Check sheet for the drawn part. Datum: minimum x, y, z corner. Units: mm. A direction names the side the tool comes from. Round coordinates to 2 decimals unless told otherwise and drop trailing zeros. Write each loop counter-clockwise with the first axis right and the second up, starting at its lowest first coordinate (ties: lowest second). Pieces come first, ordered by that corner, then holes. Notation, with made-up numbers: M 20,-15 L 79,-15 A30 cw 79,18 Z; hole C 1.5,69.5 d3. An arc over 180 degrees is marked long. One line per item, written item: value.
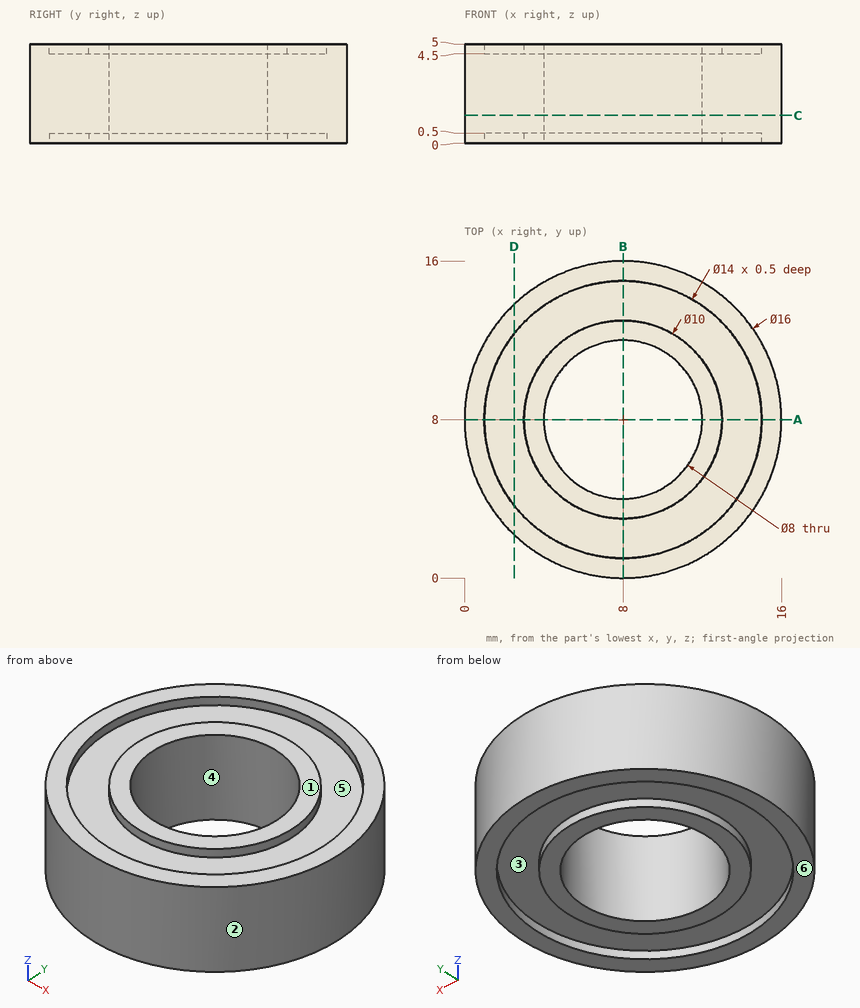
Q1. Scan lines: line 1 (Y direction, x = 8, z = 0.4); line 2 (Y direction, x = 8, z = 1.3); line 3 (X direction, y = 4.5, z = 4.1). Record each from-to range of solid material in increasing order. Write a range as [from, to].
Completed:
line 1: [0, 1], [3, 4], [12, 13], [15, 16]
line 2: [0, 4], [12, 16]
line 3: [0.81, 6.06], [9.94, 15.19]
Q2. Sectioned sample at C-C on z = 1.4. Enter the section's corners in (x, y).
Completed:
outline: C 8,8 d16; hole C 8,8 d8
Q3. Draft check along Y on the marked faces 1, 2, 3 and 4. Enter one of: pulls with the +Y half, pulls with the -Y half, needs draft (parallel to the pull), parting line crosses it, or undercut.
Completed:
face 1: needs draft
face 2: parting line crosses it
face 3: undercut
face 4: undercut
Q4. Access from +Z, -Z, +X, -X, +Y, -Y to the whole of each face (thin tool, end or side, straight path). Record for the marked faces 5 and 6.
Completed:
face 5: +Z
face 6: -Z, +X, -X, +Y, -Y
Q5. Sectioned sample at D-D on x = 2.5. Enter the section's corners in (y, z), and give its area (3 significant figures).
Completed:
outline: M 2.19,0 L 3.67,0 L 3.67,0.5 L 12.33,0.5 L 12.33,0 L 13.81,0 L 13.81,5 L 12.33,5 L 12.33,4.5 L 3.67,4.5 L 3.67,5 L 2.19,5 Z
area: 49.4 mm^2
Q6. Sectioned sample at A-A on y = 8. Enter the section's corners in (x, z).
Completed:
outline: M 0,0 L 1,0 L 1,0.5 L 3,0.5 L 3,0 L 4,0 L 4,5 L 3,5 L 3,4.5 L 1,4.5 L 1,5 L 0,5 Z; M 12,0 L 13,0 L 13,0.5 L 15,0.5 L 15,0 L 16,0 L 16,5 L 15,5 L 15,4.5 L 13,4.5 L 13,5 L 12,5 Z
Q7. Depth check by flat-ended pin: P1, Ø2, axis at x = 4.5, y = 5.5, coming from the -Z side; P2, Ø1, axis at x = 11.5, z = 2, coming from the -Y side. Enter the tip coordinate at first touch or a pass-through.
Completed:
P1: z = 0
P2: y = 0.58
